```python
from build123d import *


with BuildPart() as part:
    # Sweep1: sweep along a path in Sketch2
    with BuildLine(Plane(origin=(0, 0, 0), x_dir=(1, 0, 0), z_dir=(0, 1, 0))) as sweep1_path:
        Line((19.05, 0), (0, 0))
        Line((0, 0), (0, -19.05))
    # Sketch3 → Sweep1 (sweep)
    with BuildSketch(Plane.XY.offset(19.05)):
        Polygon((0, 0), (12.7, 0), (12.7, 6.35), (3.175, 6.35), (3.175, 19.05), (-19.05, 19.05), (-19.05, 0), (-12.7, 0), (-12.7, 12.7), (0, 12.7), align=None)
    sweep(path=sweep1_path.line, transition=Transition.RIGHT)


solid = part.part
```
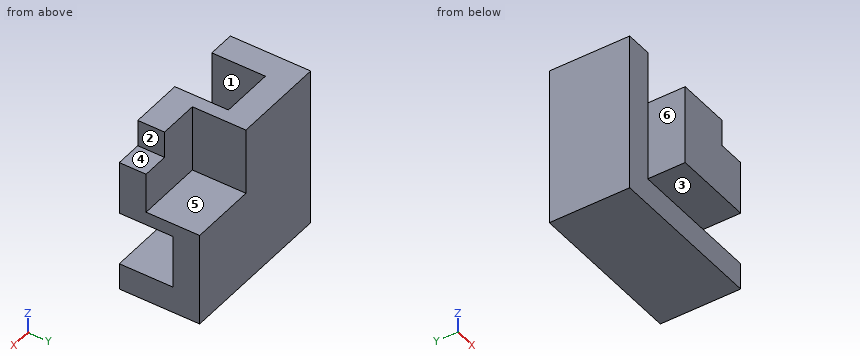
Here's how the part is built. I have some questions about the finished solid (model axes, mm). Face numbers are marked on the shaded views. A direction names the side the tool comes from. Round coordinates to 2 decimals unless told otherwise and drop trailing zeros. Loops run counter-clockwise (first coordinate to the right, second up) from the corner with the lowest first, then second, coordinate; pieces in that order, holes last.
1. If I drill on probe 1 along Z at (x, y) = (5, 6.25); probe 2 along Z at (x, y) = (6, 7) (3 decimals), over which ranges is the centre line in solid material (lowest first)?
Answers:
probe 1: z = -19.05 to -12.7, 0 to 19.05
probe 2: z = -19.05 to -12.7, 0 to 3.175
2. For the marked faces 4, 5 and 6, which set-ups out of +Z, -Z, +X, -X, +Y, -Y let a thin tool reach every point of the face, with its end or its side?
Answers:
face 4: +Z, +X, +Y, -Y
face 5: +Z, +X, +Y
face 6: +Z, -Y
3. Suppose I cut it at A-A, the plane y = 2.75. Please give me the cut outline in (x, z), and give its area (3 significant figures).
Answers:
outline: (-19.05, -19.05) - (19.05, -19.05) - (19.05, -12.7) - (-12.7, -12.7) - (-12.7, 19.05) - (-19.05, 19.05) - close; (0, 0) - (19.05, 0) - (19.05, 12.7) - (12.7, 12.7) - (12.7, 19.05) - (0, 19.05) - close
area: 766 mm2
4. Suppose I cut it at B-B, the plane z = 9. Please give me the cut outline in (x, y) (3 decimals), and give its area (3 significant figures).
Answers:
outline: (-19.05, 0) - (-12.7, 0) - (-12.7, 12.7) - (0, 12.7) - (0, 0) - (19.05, 0) - (19.05, 6.35) - (3.175, 6.35) - (3.175, 19.05) - (-19.05, 19.05) - close
area: 363 mm2
5. Will these pins go through, and if not, where does the flat tip stop? pin 1 (3 mm diameter, centred on y = 4, z = 16, fed in from +X); pin 2 (4 mm diameter, centred on x = 5.5, z = 10.5, fed in from +Y); pin 3 (12.5 mm diameter, centred on x = 9.5, z = 9, fed in from +Y); pin 4 (3 mm diameter, centred on x = 15, y = 4, fed in from +Z).
Answers:
pin 1: stops at x = 12.7
pin 2: stops at y = 6.35
pin 3: stops at y = 19.05
pin 4: stops at z = 12.7
6. Suppose I cut it at C-C, the plane x = 0.5. Please give me the cut outline in (y, z).
Answers:
outline: (0, -19.05) - (19.05, -19.05) - (19.05, 19.05) - (0, 19.05) - (0, 0) - (12.7, 0) - (12.7, -12.7) - (0, -12.7) - close
7. Thinking about a two-plate mould opening in X: for the marked faces 1, 2 and 3, which applies, released by +X, released by -X, zero draft, split by the parting line, or undercut?
Answers:
face 1: undercut
face 2: released by +X
face 3: zero draft
8. Suppose I cut it at D-D, the plane y = 12. Please give me the cut outline in (x, z) (3 decimals).
Answers:
outline: (-19.05, -19.05) - (19.05, -19.05) - (19.05, -12.7) - (-12.7, -12.7) - (-12.7, 19.05) - (-19.05, 19.05) - close; (0, 0) - (19.05, 0) - (19.05, 3.175) - (3.175, 3.175) - (3.175, 19.05) - (0, 19.05) - close
